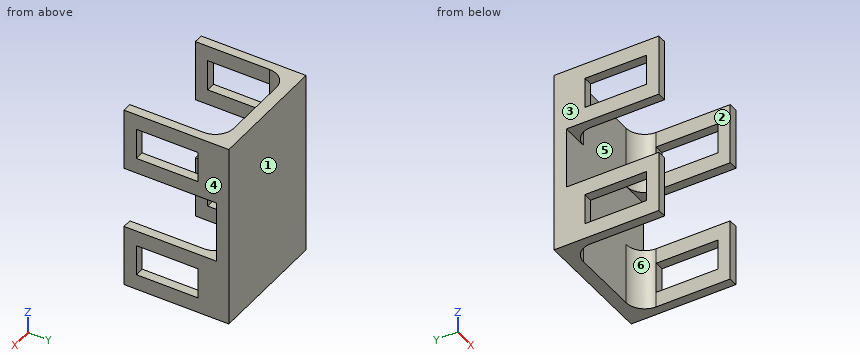
Autodesk Inventor part; units mm, degrees
ref_plane "YZ Plane" through (0, 0, 0) normal (1, 0, 0) x (0, 1, 0)
ref_plane "XZ Plane" through (0, 0, 0) normal (0, 1, 0) x (-1, 0, 0)
ref_plane "XY Plane" through (0, 0, 0) normal (0, 0, 1) x (1, 0, 0)
sketch "スケッチ1" plane through (0, 0, 0) normal (0, 0, 1) x (1, 0, 0)
  line L0 (-10, 17) -> (0, 17)
  line L1 (0, 17) -> (0, 15)
  line L2 (0, 15) -> (-10, 15)
  line L3 (-10, 15) -> (-10, 17)
  line L4 (0, -3.4) -> (0, 20.4)
  point P0 (0, 0)
  dimension "d0" = 10
  dimension "d1" = 2
  dimension "d2" = 15
extrude "押し出し1" add sketch "スケッチ1" along normal blind 5
sketch "スケッチ2" plane through (0, 0, 5) normal (0, 0, 1) x (1, 0, 0)
  line L0 (0, 17) -> (-10, 17)
  line L1 (-10, 17) -> (-8.5, 17)
  line L2 (-8.5, 17) -> (-8.5, 0)
  line L3 (-8.5, 0) -> (-10, 0)
  line L4 (-10, 0) -> (-10, 17)
  line L5 (-10, 15) -> (0, 15)
  line L6 (0, 15) -> (0, 17)
  line L7 (0, 17) -> (-10, 17)
  line L8 (-10, 17) -> (-10, 15)
  point P0 (0, 0)
  point P1 (-8.5, 15)
  dimension "d5" = 1.5
extrude "押し出し2" add sketch "スケッチ2" along normal blind 10
sketch "スケッチ3" plane through (-8.5, 0, 5) normal (1, 0, 0) x (0, 0, -1)
  line L0 (-7.5, 12) -> (-2.5, 12)
  line L1 (-2.5, 12) -> (-2.5, 2)
  line L2 (-2.5, 2) -> (-7.5, 2)
  line L3 (-7.5, 2) -> (-7.5, 12)
  line L4 (0, 0) -> (-10, 0)
  line L5 (0, 15) -> (-10, 15)
  point P0 (5, 0)
  point P1 (-5, 2)
  point P2 (-5, 0)
  dimension "d8" = 2
  dimension "d9" = 5
  dimension "d13" = 3
extrude "押し出し3" cut sketch "スケッチ3" against normal through all
fillet "フィレット1" radius 3 1 edges at (-8.5, 15, 10)
mirror "ミラー1" about plane through (0, 15, 0) normal (1, 0, 0)
mirror "ミラー2" about plane through (-5, 16, 0) normal (0, 0, -1)
properties part number "connetcor_female"
Geometry: final body of the model. Coordinates: model frame, mm. Face numbers are marked on the shaded views. A direction names the side the tool comes from. Give positions to 0.01 mm unless a question says otherwise; leave off trailing zeros. Write each loop counter-clockwise with the first axis right and the second up, starting at its lowest first coordinate (ties: lowest second). Pieces come first, ordered by that corner, then holes. Notation, with made-up numbers: (31, 80) - (36, 80) arc R21 ccw to (36, 100) - close; hole circle Ø11 at (36, 77). An arc over 180 degrees is marked (long way). Return JSON: item names as keys, results as strings. Group by question number.
1) Section C-C on y = 13.75. Return the cut outline in (x, z), plus the area to 3 significant figures.
2) Set-up query: the marked faces 4, 5 and 6. Return all of +Z, -Z, +X, -X, +Y, -Y with unobstructed straight access to the full face (end or side cutting, diameter ignored); none if empty.
3) Section A-A on y = 7.25. State how many separate pieces and enclosed holes the cut face has, plus the area to 3 significant figures.
4) Section D-D on z = -7. Return the cut outline in (x, y).
5) Line query: line 1 (X direction, y = 6.75, z = -13.5); line 2 (Y direction, x = 0.5, z = -7.25); line 3 (X direction, y = 13.5, z = -5.25). Output: solid intervals per line, ascending.
6) Mould query, pull axis X, two halves, no side actions, for the marked faces 1, 2 and 3. Classes: released by +X, released by -X, zero draft, split by the parting line, or undercut.
Filled in:
{
 "1": {"outline": "(-10, -15) - (-7.94, -15) - (-7.94, -5) - (-10, -5) - close; (-10, 5) - (-7.94, 5) - (-7.94, 15) - (-10, 15) - close; (7.94, -15) - (10, -15) - (10, -5) - (7.94, -5) - close; (7.94, 5) - (10, 5) - (10, 15) - (7.94, 15) - close", "area": "82.5 mm^2"},
 "2": {"face 4": "+Z, -Z, +X, +Y, -Y", "face 5": "-Y", "face 6": "+Z, -Z, -Y"},
 "3": {"separate pieces": "8", "enclosed holes": "0", "area": "30.0 mm^2"},
 "4": {"outline": "(-10, 0) - (-8.5, 0) - (-8.5, 12) arc R3 cw to (-5.5, 15) - (5.5, 15) arc R3 cw to (8.5, 12) - (8.5, 0) - (10, 0) - (10, 17) - (-10, 17) - close"},
 "5": {"line 1": "x = -10 to -8.5, 8.5 to 10", "line 2": "y = 15 to 17", "line 3": "x = -10 to -8.1, 8.1 to 10"},
 "6": {"face 1": "zero draft", "face 2": "undercut", "face 3": "released by -X"}
}
